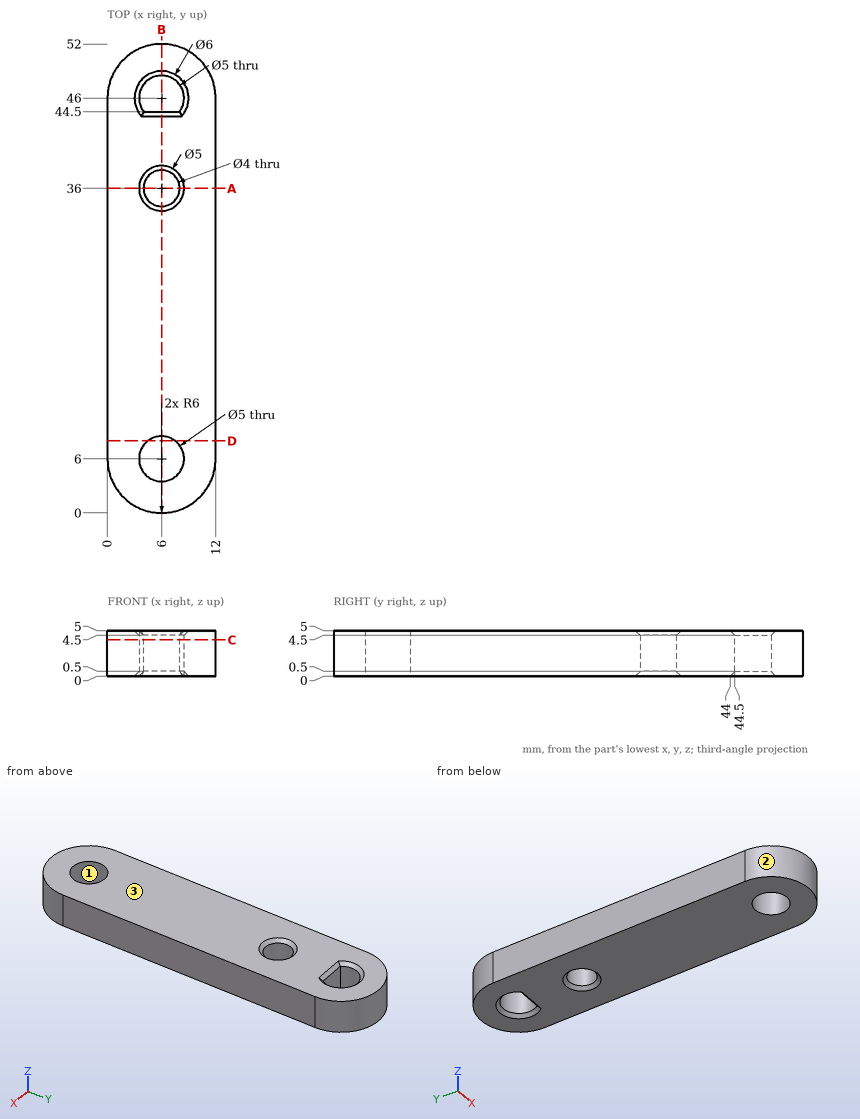
The figure shows three views and two pictorial views of one solid part (mm, origin at its lowest corner). Answer the questions. Round coordinates to 2 decimals unless told otherwise and drop trailing zeros. Loops run counter-clockwise (first coordinate to the right, second up) from the corner with the lowest first, then second, coordinate; pieces in that order, holes last. Notation, with made-up numbers: (56.5, 51) -> (66.5, 51) arc R23 cw to (66.5, 69) -> close; hole circle Ø10 at (51, 16.5). An arc over 180 degrees is marked (long way). Use one line per item in the form item = value.
(1) Find section C-C on z = 4. Give the vertices of the cut face in (x, y).
Answer list:
outline = (0, 6) arc R6 ccw to (12, 6) -> (12, 46) arc R6 ccw to (0, 46) -> close; hole circle Ø5 at (6, 6); hole circle Ø4 at (6, 36); hole (4, 44.5) -> (8, 44.5) arc R2.5 ccw (long way) to start
(2) Find section A-A on y = 36. Give the vertices of the cut face in (x, z).
Answer list:
outline = (0, 0) -> (3.5, 0) -> (4, 0.5) -> (4, 4.5) -> (3.5, 5) -> (0, 5) -> close; (8, 0.5) -> (8.5, 0) -> (12, 0) -> (12, 5) -> (8.5, 5) -> (8, 4.5) -> close
(3) For a pull along X with two mould halves and no side action, classify the marked faces 1, 2 and 3 as released by +X, released by -X, zero draft, split by the parting line, or undercut.
Answer list:
face_1 = undercut
face_2 = split by the parting line
face_3 = zero draft
(4) Find section B-B on x = 6. Give the vertices of the cut face in (y, z).
Answer list:
outline = (0, 0) -> (3.5, 0) -> (3.5, 5) -> (0, 5) -> close; (8.5, 0) -> (33.5, 0) -> (34, 0.5) -> (34, 4.5) -> (33.5, 5) -> (8.5, 5) -> close; (38, 0.5) -> (38.5, 0) -> (44, 0) -> (44.5, 0.5) -> (44.5, 4.5) -> (44, 5) -> (38.5, 5) -> (38, 4.5) -> close; (48.5, 0.5) -> (49, 0) -> (52, 0) -> (52, 5) -> (49, 5) -> (48.5, 4.5) -> close
(5) Straight lines are drawn through the part: line 1 (X direction, y = 46, z = 2.15); line 2 (Y direction, x = 7.75, z = 2.75); line 3 (Y direction, x = 4.5, z = 0.3) (3 decimals). For each, find the intervals that lie inside material, in ascending order.
Answer list:
line_1 = 0 to 3.5, 8.5 to 12
line_2 = 0.26 to 4.21, 7.79 to 35.03, 36.97 to 44.5, 47.79 to 51.74
line_3 = 0.191 to 4, 8 to 34.391, 37.609 to 44.3, 48.245 to 51.809
(6) A flat-ended cylindrical pin translates along its axis: P1, Ø2, axis at x = 5, z = 3.5, coming from the +Y side. Find the tip coordinate at first contact, or state that the pin passes through.
Answer list:
P1 = 52
(7) Find section D-D on y = 8. Give the vertices of the cut face in (x, z), then the cut area to 3 significant figures.
Answer list:
outline = (0, 0) -> (4.5, 0) -> (4.5, 5) -> (0, 5) -> close; (7.5, 0) -> (12, 0) -> (12, 5) -> (7.5, 5) -> close
area = 45.0 mm2
